from build123d import *

# Parameters (mm, degrees)
F1_DEPTH = 3.175
F3_DEPTH = 50.8
F4_R     = 6.35
F5_DEPTH = 50.8


# Not quite as in the source:
# - a length typed as a fraction of an inch, garbled in the dataset ("3 / 203.2 mm" for 3/8 in), is restored


with BuildPart() as f1:
    # F0 (on Top) → F1 (new body)
    with BuildSketch(Plane.XY):
        with BuildLine():
            Line((53.34, -21.8826867197), (76.2, -52.3626867197))
            ThreePointArc((76.2, -52.3626867197), (88.9, 36.5373132803), (0, 49.2373132803))
            Line((0, 49.2373132803), (22.86, 18.7573132803))
            Line((22.86, 18.7573132803), (-27.94, -19.3426867197))
            Line((-27.94, -19.3426867197), (-50.8, 11.1373132803))
            Line((-50.8, 11.1373132803), (-60.96, 3.5173132803))
            Line((-60.96, 3.5173132803), (-38.1, -26.9626867197))
            Line((-38.1, -26.9626867197), (-88.9, -65.0626867197))
            Line((-88.9, -65.0626867197), (-111.76, -34.5826867197))
            ThreePointArc((-111.76, -34.5826867197), (-124.46, -123.4826867197), (-35.56, -136.1826867197))
            Line((-35.56, -136.1826867197), (-58.42, -105.7026867197))
            Line((-58.42, -105.7026867197), (-22.9741035603, -79.11826439))
            Line((-22.9741035603, -79.11826439), (-8.1111921991, -67.971080869))
            Line((-8.1111921991, -67.971080869), (15.24, -98.0826867197))
            Line((15.24, -98.0826867197), (25.4, -90.4626867197))
            Line((25.4, -90.4626867197), (2.54, -59.9826867197))
            Line((2.54, -59.9826867197), (53.34, -21.8826867197))
        make_face()
    extrude(amount=F1_DEPTH)

    # F2 (on face) → F3 (cut)
    with BuildSketch(Plane(origin=(29.7060896255, -39.6081195006, 0), x_dir=(0.8, 0.6, 0), z_dir=(0.6, -0.8, 0))):
        with BuildLine():
            ThreePointArc((-78.7146071563, -9.525), (-83.2047352168, -20.3651280605), (-72.3646071563, -15.875))
            ThreePointArc((-72.3646071563, -15.875), (-74.2244790957, -11.3848719395), (-78.7146071563, -9.525))
        make_face()
    extrude(amount=-F3_DEPTH, mode=Mode.SUBTRACT)

    # F4 (on face) → F5 (cut)
    with BuildSketch(Plane(origin=(-0.7739103745, 1.0318804994, 0), x_dir=(-0.8, -0.6, 0), z_dir=(-0.6, 0.8, 0))):
        with Locations((2.2076120318, -15.875)):
            Circle(F4_R)
    extrude(amount=-F5_DEPTH, mode=Mode.SUBTRACT)


solid = f1.part
The listing builds one solid part. Answer for the finished solid, in the listing's coordinates (mm). A direction names the side the tool comes from. Give positions to 0.01 mm unless a question says otherwise; leave off trailing zeros. Write each loop counter-clockwise with the first axis right and the second up, starting at its lowest first coordinate (ties: lowest second). Pieces come first, ordered by that corner, then holes.
1) Section C-C (y = -12) is taken. Write down the section's boundary in (x, z) (3 decimals), and give its area (3 significant figures).
2) Section B-B (z = 0.7) is taken. Write down the section's boundary in (x, y), and give its area (3 significant figures).
3) Section D-D (x = -14) is taken. Write down the section's boundary in (y, z) (3 decimals).
4) For a pull along Y with two mould halves and no side action, classify faces 5 (the face through (64.61, -36.91, 1.57)), 6 (the face through (14.13, -75.436, 1.565)), 7 (the face through (-55.81, 7.38, 1.57)), 8 (the face through (-46.83, -121.156, 1.565)) as pulls with the +Y half, pulls with the -Y half, needs draft (parallel to the pull), parting line crosses it, or undercut.
5) Section A-A (y = -47.5) is taken. Write down the section's boundary in (x, z) (3 decimals).
6) A tool of negligible diameter and unlimited length cuts with its end or side. For faces 1 (the face through (11.27, 34.21, 1.57)), 2 (the face through (-39.21, -4.316, 1.565)), 3 (the face through (27.584, -41.199, 1.565)), 4 (the face through (3.401, -82.816, 1.565)), from which of +Z, -Z, +X, -X, +Y, -Y can it reach the whole face along a straight path? Write none if from no direction.
7) Given P1, Ø1.5, axis at y = -67, z = 2, coming from the +X side, flat-ended and moving along its own axis, determine where the tip first touches the part or whether it passes through.
8) Find the intervals of material crossed by L1, parallel to Y at x = -54.5, z = 2.05; L2, parallel to X at y = -49, z = 2.65; L3, parallel to Y at x = -49, z = 1.55, in increasing order.
Response:
1. outline: (-49.322, 0) - (-33.447, 0) - (-33.447, 3.175) - (-49.322, 3.175) - close; (-18.15, 0) - (100.736, 0) - (100.736, 3.175) - (-18.15, 3.175) - close
1. area: 428 mm2
2. outline: (-111.76, -34.58) arc R63.5 ccw to (-35.56, -136.18) - (-58.42, -105.7) - (-8.11, -67.97) - (15.24, -98.08) - (25.4, -90.46) - (2.54, -59.98) - (53.34, -21.88) - (76.2, -52.36) arc R63.5 ccw to (0, 49.24) - (22.86, 18.76) - (-27.94, -19.34) - (-50.8, 11.14) - (-60.96, 3.52) - (-38.1, -26.96) - (-88.9, -65.06) - close
2. area: 20,700 mm2
3. outline: (-72.388, 0) - (-8.888, 0) - (-8.888, 3.175) - (-72.388, 3.175) - close
4. face 5: pulls with the -Y half
4. face 6: undercut
4. face 7: pulls with the +Y half
4. face 8: undercut
5. outline: (-124.622, 0) - (-102.072, 0) - (-102.072, 3.175) - (-124.622, 3.175) - close; (-65.483, 0) - (19.184, 0) - (19.184, 3.175) - (-65.483, 3.175) - close; (72.553, 0) - (81.941, 0) - (81.941, 3.175) - (72.553, 3.175) - close
6. face 1: +Z, -Z, -X
6. face 2: +Z, -Z, +Y
6. face 3: +Z, -Z
6. face 4: +Z, -Z, -Y
7. P1: stops at x = 8.37
8. L1: y = -145.92 to -110.93, -102.76 to -39.26, -5.1 to 8.36
8. L2: x = -125.7 to -100.95, -67.48 to 17.18, 73.68 to 80.31
8. L3: y = -143.9 to -118.26, -98.64 to -35.14, -12.43 to 8.74
